```python
from build123d import *

# Parameters (mm, degrees)
F1_DEPTH = 25.4
F2_R     = 5.08
F3_R     = 5.08
F5_R     = 34.804273
F6_DEPTH = 25.4
F7_SIZE  = 5.08


with BuildPart() as f1:
    # F0 (on Front) → F1 (new body)
    with BuildSketch(Plane.XZ):
        Polygon((0, 83.670445), (0, 0), (94.367452, 0), (112.888888, 0), (112.888888, 83.670445), align=None)
    extrude(amount=F1_DEPTH)

    # F2
    f2_edges = [f1.edges().sort_by_distance(p)[0] for p in [
        (112.888888, 0, 41.835222),
        (0, 0, 41.835222),
        (56.444444, 0, 0),
        (56.444444, 0, 83.670445),
    ]]
    fillet(f2_edges, radius=F2_R)

    # F3
    f3_edges = [f1.edges().sort_by_distance(p)[0] for p in [
        (112.888888, -25.4, 41.835222),
        (56.444444, -25.4, 83.670445),
        (0, -25.4, 41.835222),
        (56.444444, -25.4, 0),
    ]]
    fillet(f3_edges, radius=F3_R)

    # F5 (on face) → F6 (join)
    with BuildSketch(Plane(origin=(0, 0, 0), x_dir=(-1, 0, 0), z_dir=(0, 1, 0))):
        with Locations((-53.028904, 42.805873)):
            Circle(F5_R)
    extrude(amount=F6_DEPTH)

    # F7
    f7_edges = [f1.edges().sort_by_distance(p)[0] for p in [
        (87.833177, 25.4, 42.805873),
    ]]
    chamfer(f7_edges, length=F7_SIZE)


solid = f1.part
```
Can you work these out from the model? Positions are in its coordinate system, mm. A direction names the side the tool comes from. Give positions to 0.01 mm unless a question says otherwise; leave off trailing zeros. Loops run counter-clockwise (first coordinate to the right, second up) from the corner with the lowest first, then second, coordinate; pieces in that order, holes last. Notation, with made-up numbers: M 51.5,-30.75 L 89.5,-30.75 A23 ccw 89.5,-15.75 Z; hole C 87.25,3.5 d10. An arc over 180 degrees is marked long. Use one line per item in the form item = value. Start each with the question number.
(1) On a 3-axis mill with a long thin cutter (end or side, diameter ignored), from which of +Z, -Z, +X, -X, +Y, -Y can I reach the whole of each face in a straight line? I mean faces 1 (the cylindrical face through (57.235, -1.528, 1.449)), 2 (the flat face through (90, 0, 42)). Say none if no direction works.
(2) Please list where these lines run through material, in increasing order: line 1 (Y direction, x = 15.5, z = 75.5); line 2 (X direction, y = -4, z = 67); line 3 (X direction, y = 17.5, z = 29.5).
(3) I want a section at C-C, the plane y = 22. Write out the boundary of the cut face in (x, z).
(4) I want a section at A-A, the plane x = 96. Write out the boundary of the cut face in (y, z).
(5) I'm going to push flat-ended pins straight in: P1, Ø12, axis at x = 21.5, y = 14.5, coming from the -Z side; P2, Ø8, axis at y = 1, z = 26, coming from the +X side; P3, Ø1, axis at y = 18, z = 20.5, coming from the -X side. Where does each tip first touch, or does it pass through?
(6) I want a section at B-B, the plane y = 15.5. Write out the boundary of the cut face in (x, z).
Worked out:
q1.face_1 = -Z, +X, -X, +Y
q1.face_2 = +Y
q2.line_1 = -25.4 to 0
q2.line_2 = 0.12 to 112.77
q2.line_3 = 20.87 to 85.19
q3.outline = C 53.03,42.81 d66.25
q4.outline = M -25.4,5.08 A5.08 ccw -20.32,0 L -5.08,0 A5.08 ccw 0,5.08 L 0,78.59 A5.08 ccw -5.08,83.67 L -20.32,83.67 A5.08 ccw -25.4,78.59 Z
q5.P1 = 19.15
q5.P2 = 112.44
q5.P3 = 25.9
q6.outline = C 53.03,42.81 d69.61
